from build123d import *

# Parameters (mm, degrees)
EXTRUDE_3_DEPTH      = 10
EXTRUDE_3_DEPTH_BACK = 10
FILLET_3_R           = 1.5
SKETCH_6_W           = 17
SKETCH_6_H           = 17
CUT_EXTRUDE_2_DEPTH  = 2
SKETCH_9_W           = 6
SKETCH_9_H           = 1.5
EXTRUDE_6_DEPTH      = 3
EXTRUDE_7_DEPTH      = 8
FILLET_4_R           = 1


with BuildPart() as part:
    # Sketch 3 → Extrude 3 (new body, two sides)
    with BuildSketch(Plane.XY) as extrude_3_sk:
        with BuildLine():
            Line((0.5, -10), (2, -10))
            Line((2, -10), (2, 10))
            Line((2, 10), (0.5, 10))
            ThreePointArc((0.5, 10), (-1.267766953, 9.267766953), (-2, 7.5))
            Line((-2, 7.5), (-2, -7.5))
            ThreePointArc((-2, -7.5), (-1.267766953, -9.267766953), (0.5, -10))
        make_face()
    extrude(amount=EXTRUDE_3_DEPTH)
    extrude(extrude_3_sk.sketch, amount=-EXTRUDE_3_DEPTH_BACK)

    # Fillet 3
    fillet_3_edges = [part.edges().sort_by_distance(p)[0] for p in [
        (-1.267766953, 9.267766953, -10),
        (-2, 0, -10),
        (1.25, 10, 10),
        (-1.267766953, 9.267766953, 10),
        (-2, 0, 10),
        (-1.267766953, -9.267766953, 10),
        (1.25, -10, 10),
        (-1.267766953, -9.267766953, -10),
        (1.25, -10, -10),
        (1.25, 10, -10),
    ]]
    fillet(fillet_3_edges, radius=FILLET_3_R)

    # Sketch 6 → Cut-Extrude 2 (cut)
    with BuildSketch(Plane(origin=(2, 0, 0), x_dir=(0, 0, -1), z_dir=(1, 0, 0))):
        Rectangle(SKETCH_6_W, SKETCH_6_H)
    extrude(amount=-CUT_EXTRUDE_2_DEPTH, mode=Mode.SUBTRACT)

    # Sketch 9 → Extrude 6 (add)
    with BuildSketch(Plane(origin=(2, 0, 0), x_dir=(0, 0, -1), z_dir=(1, 0, 0))):
        with Locations((0, -9.25)):
            Rectangle(SKETCH_9_W, SKETCH_9_H)
    extrude(amount=EXTRUDE_6_DEPTH)

    # Sketch 10 → Extrude 7 (add)
    with BuildSketch(Plane(origin=(0, 0, 0), x_dir=(0, 0, -1), z_dir=(1, 0, 0))):
        with BuildLine():
            Line((-0.5, 2.653299832), (-0.5, 1.090871211))
            ThreePointArc((-0.5, 1.090871211), (-0.848528137, 0.848528137), (-1.090871211, 0.5))
            Line((-1.090871211, 0.5), (-2.653299832, 0.5))
            ThreePointArc((-2.653299832, 0.5), (-1.909188309, 1.909188309), (-0.5, 2.653299832))
        make_face()
        with BuildLine():
            Line((0.5, 2.653299832), (0.5, 1.090871211))
            ThreePointArc((0.5, 1.090871211), (0.848528137, 0.848528137), (1.090871211, 0.5))
            Line((1.090871211, 0.5), (2.653299832, 0.5))
            ThreePointArc((2.653299832, 0.5), (1.909188309, 1.909188309), (0.5, 2.653299832))
        make_face()
        with BuildLine():
            Line((-2.653299832, -0.5), (-1.090871211, -0.5))
            ThreePointArc((-1.090871211, -0.5), (-0.848528137, -0.848528137), (-0.5, -1.090871211))
            Line((-0.5, -1.090871211), (-0.5, -2.653299832))
            ThreePointArc((-0.5, -2.653299832), (-1.909188309, -1.909188309), (-2.653299832, -0.5))
        make_face()
        with BuildLine():
            Line((0.5, -1.090871211), (0.5, -2.653299832))
            ThreePointArc((0.5, -2.653299832), (1.909188309, -1.909188309), (2.653299832, -0.5))
            Line((2.653299832, -0.5), (1.090871211, -0.5))
            ThreePointArc((1.090871211, -0.5), (0.848528137, -0.848528137), (0.5, -1.090871211))
        make_face()
    extrude(amount=EXTRUDE_7_DEPTH)

    # Fillet 4
    fillet_4_edges = [part.edges().sort_by_distance(p)[0] for p in [
        (5, -9.25, 3),
        (5, -9.25, -3),
    ]]
    fillet(fillet_4_edges, radius=FILLET_4_R)


solid = part.part
Could you check a few things on this model? Use its own coordinates, in mm. A direction names the side the tool comes from. Round coordinates to 2 decimals unless told otherwise and drop trailing zeros. Loops run counter-clockwise (first coordinate to the right, second up) from the corner with the lowest first, then second, coordinate; pieces in that order, holes last. Notation, with made-up numbers: (50.5, 30) - (78.5, 30) arc R18 ccw to (78.5, 64) - close; hole circle Ø10 at (11.25, 8). An arc over 180 degrees is marked (long way). Write item = value, one per line.
1) On a 3-axis mill with a long thin cutter (end or side, diameter ignored), from which of +Z, -Z, +X, -X, +Y, -Y can I reach the whole of each face in a straight line? I mean faces 5 (the cylindrical face through (1.24, 9.57, 9.55)), 6 (the flat face through (3, -9, -3)), 7 (the flat face through (5, -9, 0)), 8 (the flat face through (4, 2, -0.5)), 9 (the flat face through (3, -9, 3)). Say none if no direction works.
Computed:
face_5 = +Z, +X, -X, +Y
face_6 = -Z, +X, +Y, -Y
face_7 = +Z, -Z, +X, -Y
face_8 = +X
face_9 = +Z, +X, +Y, -Y
2) Imagine slicing it at B-B (z = 4.75). Please give me the cut outline in (x, y).
Computed:
outline = (-2, -7.5) arc R2.5 ccw to (0.5, -10) - (2, -10) - (2, -8.5) - (0, -8.5) - (0, 8.5) - (2, 8.5) - (2, 10) - (0.5, 10) arc R2.5 ccw to (-2, 7.5) - close
3) Imagine slicing it at A-A (x = 1.5). Please give me the cut outline in (y, z).
Computed:
outline = (-10, -8.5) arc R1.5 ccw to (-8.5, -10) - (8.5, -10) arc R1.5 ccw to (10, -8.5) - (10, 8.5) arc R1.5 ccw to (8.5, 10) - (-8.5, 10) arc R1.5 ccw to (-10, 8.5) - close; (-2.65, -0.5) arc R2.7 ccw to (-0.5, -2.65) - (-0.5, -1.09) arc R1.2 cw to (-1.09, -0.5) - close; (-2.65, 0.5) - (-1.09, 0.5) arc R1.2 cw to (-0.5, 1.09) - (-0.5, 2.65) arc R2.7 ccw to start; (0.5, -2.65) arc R2.7 ccw to (2.65, -0.5) - (1.09, -0.5) arc R1.2 cw to (0.5, -1.09) - close; (0.5, 1.09) arc R1.2 cw to (1.09, 0.5) - (2.65, 0.5) arc R2.7 ccw to (0.5, 2.65) - close; hole (-8.5, -8.5) - (8.5, -8.5) - (8.5, 8.5) - (-8.5, 8.5) - close
4) Imagine slicing it at D-D (y = 3.5). Please give me the cut outline in (x, z), and give its area (3 significant figures).
Computed:
outline = (-2, -8.5) arc R1.5 ccw to (-0.5, -10) - (2, -10) - (2, -8.5) - (0, -8.5) - (0, 8.5) - (2, 8.5) - (2, 10) - (-0.5, 10) arc R1.5 ccw to (-2, 8.5) - close
area = 45.0 mm2
5) If we mould it in two halves opening along Z, with no side actions, what happens to faces 1 (the cylindrical face through (1.26, -9.57, -9.55)), 2 (the cylindrical face through (-1.57, -0.11, 9.55)), 3 (the flat face through (4, -0.5, 2)), 4 (the flat face through (4, -2, 0.5))? For each: pulls with the +Z half, pulls with the -Z half, needs draft (parallel to the pull), parting line crosses it, or undercut.
Computed:
face_1 = pulls with the -Z half
face_2 = pulls with the +Z half
face_3 = undercut
face_4 = undercut
6) I'm going to push flat-ended pins straight in: P1, Ø1.2, axis at x = 4, y = 1.5, coming from the +Z side; P2, Ø0.5, axis at x = 5.5, z = -2, coming from the -Y side; P3, Ø0.5, axis at x = 3, y = -1.5, coming from the +Z side; P4, Ø3, axis at x = 7, z = 5.5, coming from the -Y side. Where does each tip first touch, or does it pass through?
Computed:
P1 = 2.55
P2 = -2.06
P3 = 2.39
P4 = through
7) Imagine slicing it at C-C (x = 3). Please give me the cut outline in (y, z), and give its area (3 significant figures).
Computed:
outline = (-10, -3) - (-8.5, -3) - (-8.5, 3) - (-10, 3) - close; (-2.65, -0.5) arc R2.7 ccw to (-0.5, -2.65) - (-0.5, -1.09) arc R1.2 cw to (-1.09, -0.5) - close; (-2.65, 0.5) - (-1.09, 0.5) arc R1.2 cw to (-0.5, 1.09) - (-0.5, 2.65) arc R2.7 ccw to start; (0.5, -2.65) arc R2.7 ccw to (2.65, -0.5) - (1.09, -0.5) arc R1.2 cw to (0.5, -1.09) - close; (0.5, 1.09) arc R1.2 cw to (1.09, 0.5) - (2.65, 0.5) arc R2.7 ccw to (0.5, 2.65) - close
area = 21.3 mm2
8) I need wall thicknesses on line 1 along Y through (x, z) = (2.5, -1.5) (3 decimals); line 2 along Y through (x, z) = (1.5, -7.5); line 3 along Z through (x, y) = (1.5, -1). Which ranges of each line are inside material? Lowest first, please. Write a range as from..to.
Computed:
line_1 = -10..-8.5, -2.245..-0.5, 0.5..2.245
line_2 = -10..-8.5, 8.5..10
line_3 = -10..-8.5, -2.51..-0.66, 0.66..2.51, 8.5..10
